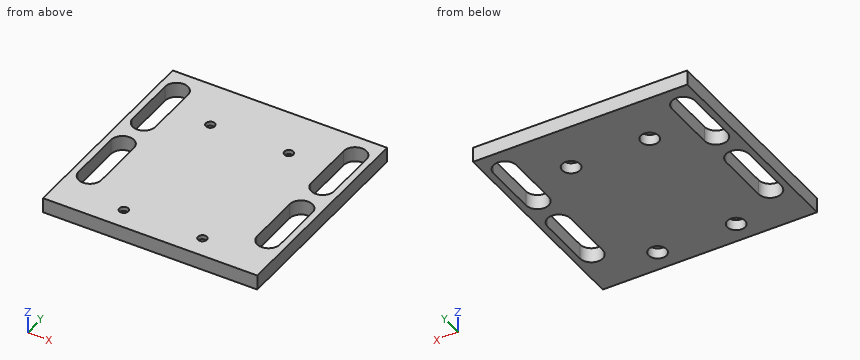
from build123d import *

# Parameters (mm, degrees)
SKETCH_1_W          = 60
SKETCH_1_H          = 60
SKETCH_1_R          = 1.25
EXTRUDE_1_DEPTH     = 4.2
SKETCH_3_R          = 2.5
CUT_EXTRUDE_2_DEPTH = 3


with BuildPart() as part:
    # 스케치1 → 보스-돌출1 (new body)
    with BuildSketch(Plane.XY):
        with Locations((0, 4)):
            Rectangle(SKETCH_1_W, SKETCH_1_H)
        with Locations((-11, 20)):
            Circle(SKETCH_1_R, mode=Mode.SUBTRACT)
        with Locations(Location((-11, -20, 0), (0, 0, 180))):
            Circle(SKETCH_1_R, mode=Mode.SUBTRACT)
        with Locations((11, -20)):
            Circle(SKETCH_1_R, mode=Mode.SUBTRACT)
        with Locations(Location((11, 20, 0), (0, 0, 180))):
            Circle(SKETCH_1_R, mode=Mode.SUBTRACT)
        with BuildLine():
            Line((-28.2, 27.5), (-28.2, 12.5))
            ThreePointArc((-28.2, 12.5), (-25, 9.3), (-21.8, 12.5))
            Line((-21.8, 12.5), (-21.8, 27.5))
            ThreePointArc((-21.8, 27.5), (-25, 30.7), (-28.2, 27.5))
        make_face(mode=Mode.SUBTRACT)
        with BuildLine():
            Line((-28.2, 2.5), (-28.2, -12.5))
            ThreePointArc((-28.2, -12.5), (-25, -15.7), (-21.8, -12.5))
            Line((-21.8, -12.5), (-21.8, 2.5))
            ThreePointArc((-21.8, 2.5), (-25, 5.7), (-28.2, 2.5))
        make_face(mode=Mode.SUBTRACT)
        with BuildLine():
            Line((21.8, 27.5), (21.8, 12.5))
            ThreePointArc((21.8, 12.5), (25, 9.3), (28.2, 12.5))
            Line((28.2, 12.5), (28.2, 27.5))
            ThreePointArc((28.2, 27.5), (25, 30.7), (21.8, 27.5))
        make_face(mode=Mode.SUBTRACT)
        with BuildLine():
            Line((21.8, 2.5), (21.8, -12.5))
            ThreePointArc((21.8, -12.5), (25, -15.7), (28.2, -12.5))
            Line((28.2, -12.5), (28.2, 2.5))
            ThreePointArc((28.2, 2.5), (25, 5.7), (21.8, 2.5))
        make_face(mode=Mode.SUBTRACT)
    extrude(amount=EXTRUDE_1_DEPTH)

    # 스케치3 → 컷-돌출2 (cut)
    with BuildSketch(Plane(origin=(0, 0, 0), x_dir=(-1, 0, 0), z_dir=(0, 0, -1))):
        with Locations((-11, 20)):
            Circle(SKETCH_3_R)
        with Locations((11, 20)):
            Circle(SKETCH_3_R)
        with Locations((-11, -20)):
            Circle(SKETCH_3_R)
        with Locations((11, -20)):
            Circle(SKETCH_3_R)
    extrude(amount=-CUT_EXTRUDE_2_DEPTH, mode=Mode.SUBTRACT)


solid = part.part
Here's how the part is built. I have some questions about the finished solid (model axes, mm). Give positions to 0.01 mm unless a question says otherwise; leave off trailing zeros. Order: outer loops, then holes, each group sorted by start corner. A loop starts at its lowest first (then second) coordinate and runs counter-clockwise, first axis right, second up. Notation, with made-up numbers: (-24, 43.5) -> (-4, 43.5) arc R24 ccw to (-4, 61.5) -> close; hole circle Ø6 at (-29, -17). An arc over 180 degrees is marked (long way). Use a Markdown table: item, result. Add a question column.
Item 1: Imagine slicing it at A-A on x = -25. Please give me the cut outline in (y, z), plus the area to 3 significant figures.
Item 2: I need wall thicknesses on line 1 (X direction, y = -4.5, z = 0.5); line 2 (Y direction, x = 11, z = 0.9); line 3 (Y direction, x = 11, z = 3.9). Which ranges of each line are inside material? Lowest first, please.
Item 3: Will this pin go through, and if not, where does the flat tip stop? pin 1 (1.5 mm diameter, centred on x = -10, y = -20, fed in from -Z).
Item 4: Imagine slicing it at B-B on z = 1.75. Give the number of separate pieces and of enclosed holes in the cut face, plus the area to 3 significant figures.
Item 5: Imagine slicing it at C-C on y = 1. Please give me the cut outline in (x, z), plus the area to 3 significant figures.
Data:
| question | item | result |
|---|---|---|
| 1 | outline | (-26, 0) -> (-15.7, 0) -> (-15.7, 4.2) -> (-26, 4.2) -> close; (5.7, 0) -> (9.3, 0) -> (9.3, 4.2) -> (5.7, 4.2) -> close; (30.7, 0) -> (34, 0) -> (34, 4.2) -> (30.7, 4.2) -> close |
| 1 | area | 72.2 mm² |
| 2 | line 1 | x = -30 to -28.2, -21.8 to 21.8, 28.2 to 30 |
| 2 | line 2 | y = -26 to -22.5, -17.5 to 17.5, 22.5 to 34 |
| 2 | line 3 | y = -26 to -21.25, -18.75 to 18.75, 21.25 to 34 |
| 3 | pin 1 | stops at z = 3 |
| 4 | separate pieces | 1 |
| 4 | enclosed holes | 8 |
| 4 | area | 3,010 mm² |
| 5 | outline | (-30, 0) -> (-28.2, 0) -> (-28.2, 4.2) -> (-30, 4.2) -> close; (-21.8, 0) -> (21.8, 0) -> (21.8, 4.2) -> (-21.8, 4.2) -> close; (28.2, 0) -> (30, 0) -> (30, 4.2) -> (28.2, 4.2) -> close |
| 5 | area | 198 mm² |
